Autodesk Inventor part; units mm, degrees
ref_plane "YZ Plane" through (0, 0, 0) normal (1, 0, 0) x (0, 1, 0)
ref_plane "XZ Plane" through (0, 0, 0) normal (0, 1, 0) x (-1, 0, 0)
ref_plane "XY Plane" through (0, 0, 0) normal (0, 0, 1) x (1, 0, 0)
sketch "Sketch1" plane through (0, 0, 0) normal (0, 0, 1) x (1, 0, 0)
  circle A0 centre (0, 0) radius 6
  line L0 (0, 2) -> (0, 34) construction
  line L1 (4, 2) -> (4, 34)
  line L2 (-4, 34) -> (-4, 2)
  arc A1 (-4, 2) -> (4, 2) centre (0, 2) ccw
  arc A2 (4, 34) -> (-4, 34) centre (0, 34) ccw
  point P0 (0, 18)
  dimension "d0" = 12
  dimension "d1" = 8
  dimension "d2" = 34
extrude "Extrusion1" add sketch "Sketch1" along normal mid plane 2.8
sketch "Sketch2" plane through (0, 0, 1.4) normal (0, 0, 1) x (1, 0, 0)
  arc A0 (4, 34) -> (-4, 34) centre (0, 34) ccw construction
  arc A1 (-4, 4.4721) -> (4, 4.4721) centre (0, 0) ccw construction
  circle A2 centre (0, 0) radius 3.5
  circle A3 centre (0, 34) radius 1.25
  line L0 (0, 15.7) -> (0, 5.7) construction
  line L1 (-1.3, 14.4) -> (-1.3, 7)
  line L2 (1.3, 7) -> (1.3, 14.4)
  arc A4 (1.3, 14.4) -> (-1.3, 14.4) centre (0, 14.4) ccw
  arc A5 (-1.3, 7) -> (1.3, 7) centre (0, 7) ccw
  point P0 (0, 10.7)
  dimension "d5" = 10
  dimension "d6" = 2.6
  dimension "d7" = 7
  dimension "d8" = 2.5
  dimension "d9" = 7
extrude "Extrusion2" cut sketch "Sketch2" against normal through all
Verification items for the finished model (mm, model axes). A direction names the side the tool comes from. Round coordinates to 2 decimals unless told otherwise and drop trailing zeros. Order: outer loops, then holes, each group sorted by start corner. A loop starts at its lowest first (then second) coordinate and runs counter-clockwise, first axis right, second up.
1) Depth check by flat-ended pin: pin 1 (1.4 mm diameter, centred on y = 12, z = 0, fed in from +X); pin 2 (1.4 mm diameter, centred on y = 20.5, z = -0.5, fed in from -X). Enter the tip coordinate at first touch or a pass-through.
Geometry says:
pin 1: stops at x = 4
pin 2: stops at x = -4
2) Material ranges on line 1 (Y direction, x = 0, z = -0.7); line 2 (X direction, y = 14, z = 0.75); line 3 (Y direction, x = -1, z = 0.3), recorded low to high.
Geometry says:
line 1: y = -6 to -3.5, 3.5 to 5.7, 15.7 to 32.75, 35.25 to 38
line 2: x = -4 to -1.3, 1.3 to 4
line 3: y = -5.92 to -3.35, 3.35 to 6.17, 15.23 to 33.25, 34.75 to 37.87
3) Tool access check on faces 5 (the flat face through (-1.3, 11, 0)), 6 (the flat face through (0, 16, -1.4)). Record the directions out of +Z, -Z, +X, -X, +Y, -Y that give a thin tool (end or side, any length) a straight path to the whole face; none if there is none.
Geometry says:
face 5: +Z, -Z
face 6: -Z, +X, -X, +Y, -Y
4) Cross-section at A-A, the plane y = 0. Record the cut outline in (x, z), plus the area to 3 significant figures.
Geometry says:
outline: (-6, -1.4) - (-3.5, -1.4) - (-3.5, 1.4) - (-6, 1.4) - close; (3.5, -1.4) - (6, -1.4) - (6, 1.4) - (3.5, 1.4) - close
area: 14.0 mm2
5) Cross-section at C-C, the plane z = -0.9. Record the cut outline in (x, y).
Geometry says:
outline: (-4, 4.47) arc R6 ccw (long way) to (4, 4.47) - (4, 34) arc R4 ccw to (-4, 34) - close; hole circle Ø7 at (0, 0); hole (-1.3, 7) arc R1.3 ccw to (1.3, 7) - (1.3, 14.4) arc R1.3 ccw to (-1.3, 14.4) - close; hole circle Ø2.5 at (0, 34)
6) Draft check along X on faces 1 (the flat face through (4, 19, 0)), 2 (the cylindrical face through (0, 15.7, 0)), 3 (the cylindrical face through (0, -6, 0)), 4 (the flat face through (-4, 19, 0)). Enter one of: +X half, -X half, draft (parallel to the pull), parting line (faces both ways), or undercut.
Geometry says:
face 1: +X half
face 2: undercut
face 3: parting line
face 4: -X half
7) Cross-section at D-D, the plane x = 1.75. Record the cut outline in (y, z), plus the area to 3 significant figures.
Geometry says:
outline: (-5.74, -1.4) - (-3.03, -1.4) - (-3.03, 1.4) - (-5.74, 1.4) - close; (3.03, -1.4) - (37.6, -1.4) - (37.6, 1.4) - (3.03, 1.4) - close
area: 104 mm2
8) Cross-section at B-B, the plane x = 0. Record the cut outline in (y, z), plus the area to 3 significant figures.
Geometry says:
outline: (-6, -1.4) - (-3.5, -1.4) - (-3.5, 1.4) - (-6, 1.4) - close; (3.5, -1.4) - (5.7, -1.4) - (5.7, 1.4) - (3.5, 1.4) - close; (15.7, -1.4) - (32.75, -1.4) - (32.75, 1.4) - (15.7, 1.4) - close; (35.25, -1.4) - (38, -1.4) - (38, 1.4) - (35.25, 1.4) - close
area: 68.6 mm2
